Verification items for the finished model (mm, model axes). Give positions to 0.01 mm unless a question says otherwise; leave off trailing zeros. Order: outer loops, then holes, each group sorted by start corner. A loop starts at its lowest first (then second) coordinate and runs counter-clockwise, first axis right, second up. Notation, with made-up numbers: (4.25, -33) -> (42.25, -33) arc R20 ccw to (42.25, -7) -> close; hole circle Ø9 at (73.25, 18.25). An arc over 180 degrees is marked (long way). Return JSON: item names as keys, results as strings. Group by question number.
(1) Cross-section at A-A on y = -3. Enter the section's corners in (x, z), then the cut area to 3 significant figures.
(2) Cross-section at C-C on x = -30. Enter the section's corners in (y, z), then the cut area to 3 significant figures.
(3) Cross-section at B-B on z = 2.3. Enter the section's corners in (x, y), then the cut area to 3 significant figures.
(4) Cross-section at D-D on y = -12.5. Enter the section's corners in (x, z), then the cut area to 3 significant figures.
(5) Thickness scan on line 1 along Y through (x, z) = (5, 3.8); line 2 along X through (y, z) = (-1, 3); line 3 along Y through (x, z) = (-0.5, 1.35). Record the ranges inside material, lowest first.
(6) Depth check by flat-ended pin: pin 1 Ø2 at (y, z) = (-16, 3) entering from -X; pin 2 Ø1.5 at (y, z) = (15.5, 1) entering from -X; pin 3 Ø6 at (x, y) = (-36, 8) entering from -Z; pin 4 Ø1.5 at (x, z) = (-26, 1) entering from +Y. Enter the tip coordinate at first touch or a pass-through.
from build123d import *

# Parameters (mm, degrees)
F1_DEPTH = 5


with BuildPart() as f1:
    # F0 (on Top) → F1 (new body)
    with BuildSketch(Plane.XY):
        with BuildLine():
            ThreePointArc((-6.74, -12.2707945953), (-14, 0), (-6.74, 12.2707945953))
            ThreePointArc((-6.74, 12.2707945953), (-11.643579322, 17.4815910795), (-17.96, 20.8431859369))
            ThreePointArc((-17.96, 20.8431859369), (-47, 0), (-17.96, -20.8431859369))
            ThreePointArc((-17.96, -20.8431859369), (-11.643579322, -17.4815910795), (-6.74, -12.2707945953))
        make_face()
        with BuildLine():
            ThreePointArc((-6.74, 12.2707945953), (-1.234276133, 13.945485378), (4.48, 13.2638455962))
            Line((4.48, 13.2638455962), (-17.96, 20.8431859369))
            ThreePointArc((-17.96, 20.8431859369), (-11.643579322, 17.4815910795), (-6.74, 12.2707945953))
        make_face()
        with BuildLine():
            ThreePointArc((-3.60125, 5.108179562), (-4.8498169631, 8.8300692851), (-6.74, 12.2707945953))
            ThreePointArc((-6.74, 12.2707945953), (-14, 0), (-6.74, -12.2707945953))
            ThreePointArc((-6.74, -12.2707945953), (-4.8498169631, -8.8300692851), (-3.60125, -5.108179562))
            ThreePointArc((-3.60125, -5.108179562), (-6.25, 0), (-3.60125, 5.108179562))
        make_face()
        with BuildLine():
            ThreePointArc((4.48, -13.2638455962), (11.3736537665, -8.1633326528), (14, 0))
            ThreePointArc((14, 0), (11.3736537665, 8.1633326528), (4.48, 13.2638455962))
            ThreePointArc((4.48, 13.2638455962), (-1.234276133, 13.945485378), (-6.74, 12.2707945953))
            ThreePointArc((-6.74, 12.2707945953), (-4.8498169631, 8.8300692851), (-3.60125, 5.108179562))
            ThreePointArc((-3.60125, 5.108179562), (2.8770373216, 5.54843728), (6.25, 0))
            ThreePointArc((6.25, 0), (2.8770373216, -5.54843728), (-3.60125, -5.108179562))
            ThreePointArc((-3.60125, -5.108179562), (-4.8498169631, -8.8300692851), (-6.74, -12.2707945953))
            ThreePointArc((-6.74, -12.2707945953), (-1.234276133, -13.945485378), (4.48, -13.2638455962))
        make_face()
        with BuildLine():
            Line((-17.96, -20.8431859369), (4.48, -13.2638455962))
            ThreePointArc((4.48, -13.2638455962), (-1.234276133, -13.945485378), (-6.74, -12.2707945953))
            ThreePointArc((-6.74, -12.2707945953), (-11.643579322, -17.4815910795), (-17.96, -20.8431859369))
        make_face()
    extrude(amount=F1_DEPTH)


solid = f1.part
Verdict:
{
 "1": {"outline": "(-46.79, 0) -> (-5.48, 0) -> (-5.48, 5) -> (-46.79, 5) -> close; (5.48, 0) -> (13.67, 0) -> (13.67, 5) -> (5.48, 5) -> close", "area": "248 mm²"},
 "2": {"outline": "(-21.42, 0) -> (21.42, 0) -> (21.42, 5) -> (-21.42, 5) -> close", "area": "214 mm²"},
 "3": {"outline": "(-17.96, -20.84) -> (4.48, -13.26) arc R14 ccw to (4.48, 13.26) -> (-17.96, 20.84) arc R22 ccw (long way) to start; hole circle Ø12.5 at (0, 0)", "area": "1,890 mm²"},
 "4": {"outline": "(-43.1, 0) -> (6.3, 0) -> (6.3, 5) -> (-43.1, 5) -> close", "area": "247 mm²"},
 "5": {"line 1": "-13.08 to -3.75, 3.75 to 13.08", "line 2": "-46.98 to -6.17, 6.17 to 13.96", "line 3": "-14.95 to -6.23, 6.23 to 14.95"},
 "6": {"pin 1": "x = -41.09", "pin 2": "x = -41.32", "pin 3": "z = 0", "pin 4": "y = 22"}
}
